Read the model definition and answer for the solid it produces. Units are mm, in the model's axes. Coordinates: 2 decimals unless noted, no trailing zeros. Loops run counter-clockwise (first coordinate to the right, second up) from the corner with the lowest first, then second, coordinate; pieces in that order, holes last.
Q1. Straight lines are drawn through the part: line 1 (Y direction, x = -3.1, z = 245.5); line 2 (Y direction, x = -0.4, z = 213.5); line 3 (Y direction, x = -2.5, z = 250). For each, find the intervals that lie inside material, in ascending order.
Q2. Flat-ended cylindrical pins translate along their axes: P1, Ø2, axis at x = -1.5, y = 695.5, coming from the -Z side; P2, Ø2, axis at x = -2, z = 211.5, coming from the +Y side; P3, Ø3, axis at y = 468, z = 233.5, coming from the +X side; P4, Ø2, axis at x = -1, z = 256, coming from the -Y side. Find the tip coordinate at first contact, or state that the pin passes through.
Q3. Section A-A (y = 299) is taken. Give the vertices of the cut face in (x, z), then the cut area to 3 significant figures.
Q4. Section B-B (y = 593) is taken. Give the vertices of the cut face in (x, z).
from build123d import *

# Parameters (mm, degrees)
F1_DEPTH = 4
F2_ANGLE = 90
F3_ANGLE = 180


with BuildPart() as f1:
    # F0 (on Right) → F1 (new body)
    with BuildSketch(Plane.YZ):
        Polygon((-4.2630598, 224.8000076), (-3.8891464, 210.6000106), (7.3218294, -304.8), (19.4630294, -304.8), (19.4630294, -229.3999984), (23.4630468, -229.3999984), (23.4630468, -189.4000022), (19.4630294, -189.4000022), (19.4630294, 170.6000144), (23.4630468, 170.6000144), (23.4630468, 210.6000106), (19.4630294, 210.6000106), (19.4630294, 304.8), (-5.9369706, 304.8), (-5.0152046, 262.3993228), (-5.482082, 260.6712084), (-6.1067696, 258.9936908), (-6.883908, 257.381121), (-7.806817, 255.847342), (-8.867648, 254.4054856), (-10.057257, 253.0678962), (-11.3654586, 251.8460546), (-12.7810514, 250.7504256), (-14.2918942, 249.7904072), (-15.885033, 248.9742036), (-17.546828, 248.3088506), (-19.2630552, 247.8000124), (-23.4630468, 247.8000124), (-23.4630468, 224.8000076), align=None)
        Polygon((-14.4949672, 233.4296322), (-15.2101042, 234.361609), (-15.6596588, 235.4469256), (-15.8129986, 241.1116082), (-15.6596588, 242.2762998), (-15.2101042, 243.3616164), (-14.4949672, 244.2935932), (-13.5629904, 245.0087302), (-12.4776738, 245.4582594), (-11.3130076, 245.6115992), (-10.148316, 245.4582594), (-9.0629994, 245.0087302), (-8.1310226, 244.2935932), (-7.4158856, 243.3616164), (-6.966331, 242.2762998), (-6.8129912, 241.1116082), (-6.8129912, 236.6116172), (-6.966331, 235.4469256), (-7.4158856, 234.361609), (-8.1310226, 233.4296322), (-9.0629994, 232.7144952), (-10.148316, 232.2649406), (-11.3130076, 232.1116008), (-12.4776738, 232.2649406), (-13.5629904, 232.7144952), align=None, mode=Mode.SUBTRACT)
    extrude(amount=F1_DEPTH)


with BuildPart() as f1_1:
    # F2: moved
    add(f1.part.rotate(Axis((2, 23.4630468, 210.6000106), (-1, 0, 0)), F2_ANGLE))


with BuildPart() as f1_2:
    # F3: moved
    add(f1_1.part.rotate(Axis((0, 117.6630362, 227.300028), (0, 0, 1)), F3_ANGLE))


solid = f1_2.part
Numbers:
1. line 1: y = 170.67 to 176.87, 190.34 to 197.66
1. line 2: y = 211.86 to 251.86, 611.86 to 651.86
1. line 3: y = 173.51 to 197.66
2. P1: stops at z = 214.6
2. P2: stops at y = 651.86
2. P3: stops at x = 0
2. P4: stops at y = 174.66
3. outline: (-4, 214.6) - (0, 214.6) - (0, 236.06) - (-4, 236.06) - close
3. area: 85.8 mm2
4. outline: (-4, 214.6) - (0, 214.6) - (0, 229.66) - (-4, 229.66) - close
